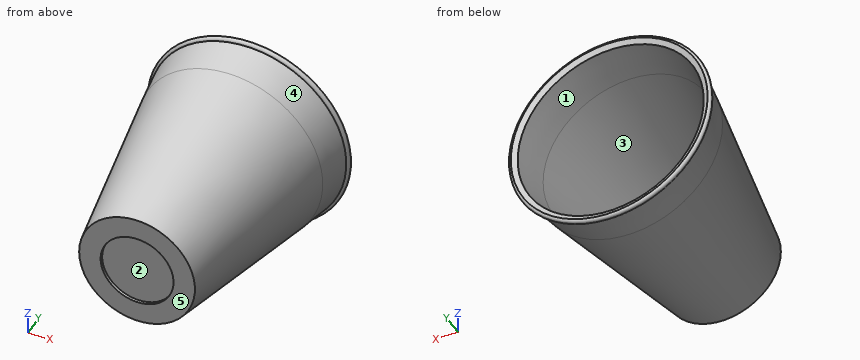
```python
from build123d import *


with BuildPart() as part:
    # Sketch1 → Revolve1 (revolve)
    with BuildSketch(Plane.XY):
        with BuildLine():
            Line((-32.130708731, -1), (-34, 0))
            ThreePointArc((-34, 0), (-35, -1), (-34, -2))
            Line((-34, -2), (-32, -14))
            Line((-32, -14), (-20, -77))
            Line((-20, -77), (-12.6, -77))
            Line((-12.6, -77), (-12.6, -75.97))
            Line((-12.6, -75.97), (0, -75.97))
            Line((0, -75.97), (0, -74))
            Line((0, -74), (-18.535470636, -74))
            Line((-18.535470636, -74), (-29.964042064, -14))
            Line((-29.964042064, -14), (-32.130708731, -1))
        make_face()
    revolve(axis=Axis((0, 0, 0), (0, -1, 0)))


solid = part.part
```
Here's how the part is built. I have some questions about the finished solid (model axes, mm). Face numbers are marked on the shaded views. A direction names the side the tool comes from. Coordinates: 2 decimals unless noted, no trailing zeros. Write each loop counter-clockwise with the first axis right and the second up, starting at its lowest first coordinate (ties: lowest second). Pieces come first, ordered by that corner, then holes. Notation, with made-up numbers: M 68,45 L 111,45 A24 ccw 111,79 Z; hole C 41.5,12 d2. An arc over 180 degrees is marked long. Answer as CSV lines item,"result". Start each with the question number.
Q1. Suppose I cut it at A-A, the plane z = 0. List the corners of the cut face in (x, y) for me, then the cut area to 3 significant figures.
Q2. Suppose I cut it at D-D, the plane y = -21.5. List the corners of the cut face in (x, z) for me, then the cut area to 3 significant figures.
Q3. Suppose I cut it at B-B, the plane x = 0. List the corners of the cut face in (y, z) for me, then the cut area to 3 significant figures.
Q4. If we mould it in two halves opening along X, with no side actions, what happens to the marked faces 3, 4 and 5? For each: pulls with the +X half, pulls with the -X half, needs draft (parallel to the pull), parting line crosses it, or undercut.
Q5. Will these pins go through, and if not, where does the flat tip stop? pin 1 Ø5 at (x, y) = (-22.5, -66) entering from +Z; pin 2 Ø5 at (x, z) = (-1, -5) entering from -Y; pin 3 Ø12 at (y, z) = (-37, 9.5) entering from +X.
Q6. I need wall thicknesses on probe 1 along Y at (x, z) = (-7, -7); probe 2 along X at (y, z) = (-76.5, 0). Which ranges of each line are inside material? Lowest first, please. Write a range as [from, to].
Q7. Suppose I cut it at C-C, the plane y = -48. List the corners of the cut face in (x, z) for me.
Q8. For the marked faces 1 and 2, which set-ups out of +Z, -Z, +X, -X, +Y, -Y let a thin tool reach every point of the face, with its end or its side?
Entries:
1,outline,"M -34,-2 L -32,-14 L -20,-77 L -12.6,-77 L -12.6,-75.97 L 12.6,-75.97 L 12.6,-77 L 20,-77 L 32,-14 L 34,-2 A1 ccw 34,0 L 32.13,-1 L 29.96,-14 L 18.54,-74 L -18.54,-74 L -29.96,-14 L -32.13,-1 L -34,0 A1 ccw Z"
1,area,"398 mm²"
2,outline,"C 0,0 d61.14; hole C 0,0 d57.07"
2,area,"378 mm²"
3,outline,"M -77,-20 L -14,-32 L -2,-34 A1 ccw 0,-34 L -1,-32.13 L -14,-29.96 L -74,-18.54 L -74,18.54 L -14,29.96 L -1,32.13 L 0,34 A1 ccw -2,34 L -14,32 L -77,20 L -77,12.6 L -75.97,12.6 L -75.97,-12.6 L -77,-12.6 Z"
3,area,"398 mm²"
4,face 3,"undercut"
4,face 4,"parting line crosses it"
4,face 5,"needs draft"
5,pin 1,"stops at z = 9.51"
5,pin 2,"stops at y = -75.97"
5,pin 3,"stops at x = 27.94"
6,probe 1,"y = [-75.97, -74]"
6,probe 2,"x = [-20.1, -12.6], [12.6, 20.1]"
7,outline,"C 0,0 d51.05; hole C 0,0 d46.98"
8,face 1,"+Y"
8,face 2,"-Y"
